from build123d import *

# Parameters (mm, degrees)
SKETCH1_R           = 10
BOSS_EXTRUDE1_DEPTH = 25.4
SKETCH2_W           = 10
SKETCH2_H           = 45.4
CUT_EXTRUDE1_DEPTH  = 116.003478208
SKETCH3_R           = 2.5
CUT_EXTRUDE2_DEPTH  = 107.255917482


with BuildPart() as part:
    # Sketch1 → Boss-Extrude1 (new body)
    with BuildSketch(Plane.XY):
        with BuildLine():
            Line((-25.4, 0), (-25.4, 100))
            Line((-25.4, 100), (25.4, 100))
            Line((25.4, 100), (25.4, 0))
            ThreePointArc((25.4, 0), (0, -25.4), (-25.4, 0))
        make_face()
        Circle(SKETCH1_R, mode=Mode.SUBTRACT)
    extrude(amount=BOSS_EXTRUDE1_DEPTH)

    # Sketch2 → Cut-Extrude1 (cut, through all)
    with BuildSketch(Plane.ZY.offset(25.4)):
        with Locations((12.7, -2.7)):
            Rectangle(SKETCH2_W, SKETCH2_H)
    extrude(amount=-CUT_EXTRUDE1_DEPTH, mode=Mode.SUBTRACT)

    # Sketch3 → Cut-Extrude2 (cut, through all)
    with BuildSketch(Plane.XY.offset(25.4)):
        with Locations((-11.25, 90)):
            Circle(SKETCH3_R)
        with Locations((11.25, 90)):
            Circle(SKETCH3_R)
        with Locations((11.25, 55)):
            Circle(SKETCH3_R)
        with Locations((-11.25, 55)):
            Circle(SKETCH3_R)
    extrude(amount=-CUT_EXTRUDE2_DEPTH, mode=Mode.SUBTRACT)


solid = part.part
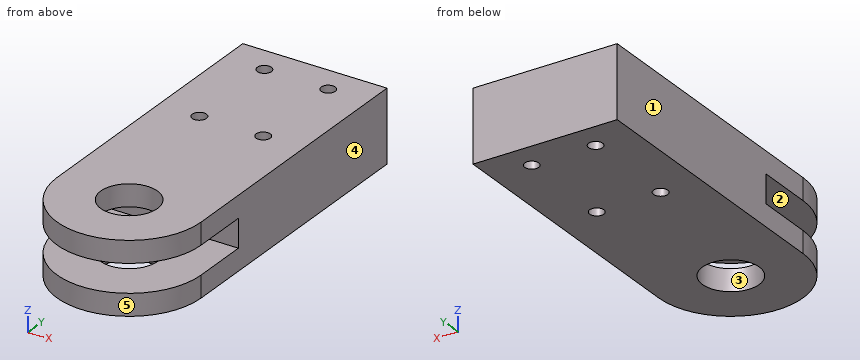
Read the model definition and answer for the solid it produces. Units are mm, in the model's axes. Face numbers are marked on the shaded views. A direction names the side the tool comes from. Round coordinates to 2 decimals unless told otherwise and drop trailing zeros. Write each loop counter-clockwise with the first axis right and the second up, starting at its lowest first coordinate (ties: lowest second). Pieces come first, ordered by that corner, then holes. Notation, with made-up numbers: (-37.5, -37) - (-17.5, -37) arc R24 ccw to (-17.5, 0) - close; hole circle Ø10 at (70, 14). An arc over 180 degrees is marked (long way). One line per question, with ' | ' between items. Start each with the question number.
1. Section C-C (y = 16) is taken. Determine the outline of the cut face in (x, z), and give its area (3 significant figures).
2. Each of these flat-tipped pins is pushed along its axis until it touches: pin 1 (1 mm diameter, centred on y = 0.5, z = 16.5, fed in from +X); pin 2 (8 mm diameter, centred on x = 1.5, z = 11.5, fed in from -Y). Where does it stop, or does it pass through?
3. Section A-A (y = 55) is taken. Determine the outline of the cut face in (x, z), and give its area (3 significant figures).
4. Section B-B (z = 23.5) is taken. Determine the outline of the cut face in (x, y).
5. For a pull along Y with two mould halves and no side action, classify the marked faces 3, 4 and 5 as +Y half, -Y half, draft (parallel to the pull), parting line (faces both ways), or undercut.
6. Section D-D (z = 10.5) is taken. Determine the outline of the cut face in (x, y), and give its area (3 significant figures).
7. Find the intervals of material crossed by probe 1 along Y at (x, z) = (11.25, 10.25); probe 2 along Z at (x, y) = (-16, -18); probe 3 along Y at (x, z) = (0, 2.25), in increasing order. Write a range as [from, to].
8. For the marked faces 1 and 2, determine the directions among +Z, -Z, +X, -X, +Y, -Y from which every point of the face is accessible in a straight line to the end or side of a thin tool.
Filled in:
1) outline: (-25.4, 0) - (25.4, 0) - (25.4, 7.7) - (-25.4, 7.7) - close; (-25.4, 17.7) - (25.4, 17.7) - (25.4, 25.4) - (-25.4, 25.4) - close | area: 782 mm²
2) pin 1: through | pin 2: y = -25.4
3) outline: (-25.4, 0) - (-13.75, 0) - (-13.75, 25.4) - (-25.4, 25.4) - close; (-8.75, 0) - (8.75, 0) - (8.75, 25.4) - (-8.75, 25.4) - close; (13.75, 0) - (25.4, 0) - (25.4, 25.4) - (13.75, 25.4) - close | area: 1,040 mm²
4) outline: (-25.4, 0) arc R25.4 ccw to (25.4, 0) - (25.4, 100) - (-25.4, 100) - close; hole circle Ø5 at (-11.25, 55); hole circle Ø5 at (-11.25, 90); hole circle Ø20 at (0, 0); hole circle Ø5 at (11.25, 55); hole circle Ø5 at (11.25, 90)
5) face 3: undercut | face 4: draft | face 5: -Y half
6) outline: (-25.4, 20) - (25.4, 20) - (25.4, 100) - (-25.4, 100) - close; hole circle Ø5 at (-11.25, 55); hole circle Ø5 at (-11.25, 90); hole circle Ø5 at (11.25, 55); hole circle Ø5 at (11.25, 90) | area: 3,990 mm²
7) probe 1: [20, 52.5], [57.5, 87.5], [92.5, 100] | probe 2: [0, 7.7], [17.7, 25.4] | probe 3: [-25.4, -10], [10, 100]
8) face 1: +Z, -Z, -X, +Y, -Y | face 2: +X, -X, -Y
